```python
from build123d import *

# Parameters (mm, degrees)
ESQUISSE1_R             = 22
ESQUISSE1_R_2           = 1.5
BOSS_EXTRU_1_DEPTH      = 6
ESQUISSE2_R             = 16.25
ESQUISSE2_R_2           = 6.9
ENL_V_MAT_EXTRU_1_DEPTH = 3.3
ENL_V_MAT_EXTRU_2_DEPTH = 3


with BuildPart() as part:
    # Esquisse1 → Boss.-Extru.1 (new body)
    with BuildSketch(Plane(origin=(0, 0, 0), x_dir=(1, 0, 0), z_dir=(0, 1, 0))):
        Circle(ESQUISSE1_R)
        with Locations((-3.5, 0)):
            Circle(ESQUISSE1_R_2, mode=Mode.SUBTRACT)
        with Locations((3.5, 0)):
            Circle(ESQUISSE1_R_2, mode=Mode.SUBTRACT)
    extrude(amount=BOSS_EXTRU_1_DEPTH)

    # Esquisse2 → Enlèv. mat.-Extru.1 (cut)
    with BuildSketch(Plane.XZ):
        Circle(ESQUISSE2_R)
        Circle(ESQUISSE2_R_2, mode=Mode.SUBTRACT)
    extrude(amount=-ENL_V_MAT_EXTRU_1_DEPTH, mode=Mode.SUBTRACT)

    # Esquisse3 → Enlèv. mat.-Extru.2 (cut)
    with BuildSketch(Plane(origin=(0, 3.3, 0), x_dir=(-1, 0, 0), z_dir=(0, -1, 0))):
        with BuildLine():
            Line((-13.940625792, -4.008679646), (-13.940625792, 4.008679646))
            ThreePointArc((-13.940625792, 4.008679646), (-11.846146155, 6.103159283), (-9.751666518, 4.008679646))
            Line((-9.751666518, 4.008679646), (-9.751666518, -4.008679646))
            ThreePointArc((-9.751666518, -4.008679646), (-11.846146155, -6.103159283), (-13.940625792, -4.008679646))
        make_face()
    extrude(amount=-ENL_V_MAT_EXTRU_2_DEPTH, mode=Mode.SUBTRACT)


solid = part.part
```
CAD build for the part. Positions are in the model's coordinates, mm. A direction names the side the tool comes from. Coordinates: 2 decimals unless noted, no trailing zeros. Order: outer loops, then holes, each group sorted by start corner. A loop starts at its lowest first (then second) coordinate and runs counter-clockwise, first axis right, second up. Notation, with made-up numbers: (19, 39.5) - (44, 39.5) arc R8 cw to (44, 53.5) - close; hole circle Ø1 at (-8, 30). An arc over 180 degrees is marked (long way). Use a Markdown table: item, result. Add a question column.
(1) Drill centre lines: line 1 along X through (y, z) = (4.15, 0); line 2 along Z through (x, y) = (0, 1.7); line 3 along X through (y, z) = (1.7, -2). Where is each one in solid material? Low to high. Write a range as [from, to].
(2) Saw through at D-D (z = 5.5). Give the cut face in (x, y), then the cut area to 3 significant figures.
(3) Saw through at A-A (y = 4.75). Give the cut face in (x, z), then the cut area to 3 significant figures.
(4) Saw through at B-B (z = 0). Give the cut face in (x, y), then the cut area to 3 significant figures.
(5) Which spindle directions (+Z, -Z, +X, -X, +Y, -Y) get a long thin tool onto all of the face, cutting with end or side? Do faces 5 (the face through (0, 0, 0)), 6 (the face through (11.8, 4.631, 6.103)), 7 (the face through (15.5, 1.63, 4.88)). Say none if no direction does.
(6) Pull direction X, two halves, no side cores. Call faces 1 (the face through (-0.9, 1.63, 6.84)), 2 (the face through (-10, 0, 13)), 3 (the face through (-7.4, 3.3, 0.2)), 4 (the face through (-4.769, 2.958, 21.477)): +X half, -X half, draft (parallel to the pull), parting line (faces both ways), or undercut.
(7) Flat gauge pins, fed straight in: pin 1 (6 mm diameter, centred on x = -2, z = -2.5, fed in from -Y); pin 2 (3 mm diameter, centred on y = 5, z = 2, fed in from -X). Where does each tip first touch, or does it go through?
(8) Saw through at C-C (x = -3.5). Give the cut face in (y, z), then the cut area to 3 significant figures.
Solved:
| question | item | result |
|---|---|---|
| 1 | line 1 | x = [-22, -5], [-2, 2], [5, 9.75], [13.94, 22] |
| 1 | line 2 | z = [-22, -16.25], [-6.9, 6.9], [16.25, 22] |
| 1 | line 3 | x = [-21.91, -16.13], [-6.6, 6.6], [16.13, 21.91] |
| 2 | outline | (-21.3, 0) - (-15.29, 0) - (-15.29, 3.3) - (-4.17, 3.3) - (-4.17, 0) - (4.17, 0) - (4.17, 3.3) - (10.38, 3.3) - (10.38, 6) - (-21.3, 6) - close; (13.32, 3.3) - (15.29, 3.3) - (15.29, 0) - (21.3, 0) - (21.3, 6) - (13.32, 6) - close |
| 2 | area | 174 mm² |
| 3 | outline | circle Ø44 at (0, 0); hole circle Ø3 at (-3.5, 0); hole circle Ø3 at (3.5, 0); hole (9.75, -4.01) arc R2.09 ccw to (13.94, -4.01) - (13.94, 4.01) arc R2.09 ccw to (9.75, 4.01) - close |
| 3 | area | 1,460 mm² |
| 4 | outline | (-22, 0) - (-16.25, 0) - (-16.25, 3.3) - (-6.9, 3.3) - (-6.9, 0) - (-5, 0) - (-5, 6) - (-22, 6) - close; (-2, 0) - (2, 0) - (2, 6) - (-2, 6) - close; (5, 0) - (6.9, 0) - (6.9, 3.3) - (9.75, 3.3) - (9.75, 6) - (5, 6) - close; (13.94, 3.3) - (16.25, 3.3) - (16.25, 0) - (22, 0) - (22, 6) - (13.94, 6) - close |
| 4 | area | 155 mm² |
| 5 | face 5 | +Z, -Z, +X, -X, -Y |
| 5 | face 6 | +Y, -Y |
| 5 | face 7 | -Y |
| 6 | face 1 | undercut |
| 6 | face 2 | draft |
| 6 | face 3 | undercut |
| 6 | face 4 | parting line |
| 7 | pin 1 | stops at y = 0 |
| 7 | pin 2 | stops at x = -21.99 |
| 8 | outline | (0, -21.72) - (6, -21.72) - (6, -1.5) - (0, -1.5) - (0, -5.95) - (3.3, -5.95) - (3.3, -15.87) - (0, -15.87) - close; (0, 1.5) - (6, 1.5) - (6, 21.72) - (0, 21.72) - (0, 15.87) - (3.3, 15.87) - (3.3, 5.95) - (0, 5.95) - close |
| 8 | area | 177 mm² |
